from build123d import *

# Parameters (mm, degrees)
ODEBRAT_VYSUNUT_M2_DEPTH      = 84.740671122
ODEBRAT_VYSUNUT_M2_DEPTH_BACK = 84.740671122
SKICA4_R                      = 2.1
ODEBRAT_VYSUNUT_M3_DEPTH      = 84.740671122
ODEBRAT_VYSUNUT_M3_DEPTH_BACK = 46
SKICA6_R                      = 4
ZKOSEN_1_SIZE                 = 0.5


with BuildPart() as part:
    # Skica1 → Rotovat1 (revolve)
    with BuildSketch(Plane.XY, mode=Mode.PRIVATE) as rotovat1_sk:
        Polygon((0, 0), (32.5, 0), (32.5, 5), (7.5, 70), (0, 70), align=None)
    revolve(rotovat1_sk.sketch.rotate(Axis((0, 0, 0), (0, -1, 0)), 90), axis=Axis((0, 0, 0), (0, -1, 0)))

    # Skica4 → Odebrat vysunutím2 (cut, two sides: drawn at the far end of the back side and taken through both)
    with BuildSketch(Plane(origin=(0, 70, 0), x_dir=(1, 0, 0), z_dir=(0, 1, 0)).offset(-ODEBRAT_VYSUNUT_M2_DEPTH_BACK)):
        with Locations(Location((0, 0, 0), (0, 0, 270))):
            Circle(SKICA4_R)
    extrude(amount=ODEBRAT_VYSUNUT_M2_DEPTH + ODEBRAT_VYSUNUT_M2_DEPTH_BACK, mode=Mode.SUBTRACT)

    # Skica6 → Odebrat vysunutím3 (cut, two sides: drawn at the far end of the back side and taken through both)
    with BuildSketch(Plane(origin=(0, 70, 0), x_dir=(1, 0, 0), z_dir=(0, 1, 0)).offset(-ODEBRAT_VYSUNUT_M3_DEPTH_BACK)):
        with Locations(Location((0, 0, 0), (0, 0, 90))):
            Circle(SKICA6_R)
    extrude(amount=ODEBRAT_VYSUNUT_M3_DEPTH + ODEBRAT_VYSUNUT_M3_DEPTH_BACK, mode=Mode.SUBTRACT)

    # Zkosení1
    zkosen_1_edges = [part.edges().sort_by_distance(p)[0] for p in [
        (0, 24, -2.1),
    ]]
    chamfer(zkosen_1_edges, length=ZKOSEN_1_SIZE)


solid = part.part
Check sheet for the modelled part. Datum: model origin and axes. Units: mm. A direction names the side the tool comes from. Round coordinates to 2 decimals unless told otherwise and drop trailing zeros. Write each loop counter-clockwise with the first axis right and the second up, starting at its lowest first coordinate (ties: lowest second). Pieces come first, ordered by that corner, then holes. Notation, with made-up numbers: (73, 75.5) -> (114, 75.5) arc R22 ccw to (114, 105.5) -> close; hole circle Ø3 at (44, 73.25). An arc over 180 degrees is marked (long way). Answer as CSV lines item,"result". Start each with the question number.
1) Section check D-D on y = 7. Enter the section's corners in (x, z), and give its area (3 significant figures).
2) Release check for a two-part mould opening along Z. For faces 1 (the cylindrical face through (3.905, 46.678, 0.867)), 2 (the flat face through (3, 70, 3)), 3 (the cylindrical face through (-9.76, 2.54, 31)) record: pulls with the +Z half, pulls with the -Z half, needs draft (parallel to the pull), parting line crosses it, or undercut.
3) Material ranges on line 1 (X direction, y = 47, z = 0); line 2 (Z direction, x = -6, y = 64.5); line 3 (X direction, y = 10, z = 0), recorded low to high. Write a range as from..to.
4) Go/stop test with flat-tipped pins: P1, Ø4, axis at x = 22, y = 26.5, coming from the -Z side; P2, Ø4, axis at x = 1, z = 1.5, coming from the +Y side; P3, Ø1.5, axis at y = 29.5, z = 5, coming from the -X side. Record where each tip stops, or that it passes through.
5) Section check B-B on x = 0. Enter the section's corners in (y, z).
6) Tool access check on faces 4 (the flat face through (0, 0, -7)), 5 (the flat face through (0, 24, -3)). Record the directions out of +Z, -Z, +X, -X, +Y, -Y that give a thin tool (end or side, any length) a straight path to the whole face; none if there is none.
7) Section check C-C on y = 47. Enter the section's corners in (x, z).
8) Section check A-A on z = 0. Enter the section's corners in (x, y).
Found:
1,outline,"circle Ø63.46 at (0, 0); hole circle Ø4.2 at (0, 0)"
1,area,"3,150 mm^2"
2,face 1,"undercut"
2,face 2,"needs draft"
2,face 3,"parting line crosses it"
3,line 1,"x = -16.35..-4, 4..16.35"
3,line 2,"z = -7.51..7.51"
3,line 3,"x = -30.58..-2.1, 2.1..30.58"
4,P1,"stops at z = -13.98"
4,P2,"stops at y = 24"
4,P3,"stops at x = -22.86"
5,outline,"(0, -32.5) -> (5, -32.5) -> (70, -7.5) -> (70, -4) -> (24, -4) -> (24, -2.6) -> (23.5, -2.1) -> (0, -2.1) -> close; (0, 2.1) -> (23.5, 2.1) -> (24, 2.6) -> (24, 4) -> (70, 4) -> (70, 7.5) -> (5, 32.5) -> (0, 32.5) -> close"
6,face 4,"+Z, -Z, +X, -X, -Y"
6,face 5,"+Y"
7,outline,"circle Ø32.69 at (0, 0); hole circle Ø8 at (0, 0)"
8,outline,"(-32.5, 0) -> (-2.1, 0) -> (-2.1, 23.5) -> (-2.6, 24) -> (-4, 24) -> (-4, 70) -> (-7.5, 70) -> (-32.5, 5) -> close; (2.1, 0) -> (32.5, 0) -> (32.5, 5) -> (7.5, 70) -> (4, 70) -> (4, 24) -> (2.6, 24) -> (2.1, 23.5) -> close"
